For this review, take the finished solid that the model builds, in its own axes (mm). Face numbers are marked on the shaded views. A direction names the side the tool comes from. Give positions to 0.01 mm unless a question says otherwise; leave off trailing zeros. Order: outer loops, then holes, each group sorted by start corner. A loop starts at its lowest first (then second) coordinate and runs counter-clockwise, first axis right, second up. Notation, with made-up numbers: (-33, 82.5) - (3, 82.5) arc R20 cw to (3, 109.5) - close; hole circle Ø9 at (-16.75, 3). An arc over 180 degrees is marked (long way). One line per item, written item: value.
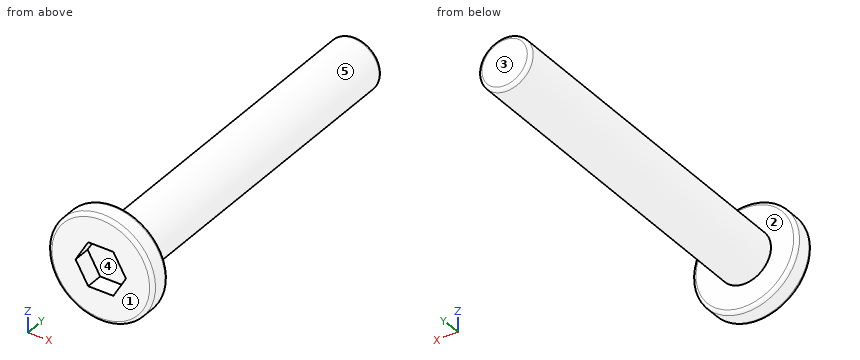
```python
from build123d import *

# Parameters (mm, degrees)
FILLET1_R          = 0.2
CUT_EXTRUDE1_DEPTH = 1


with BuildPart() as part:
    # Sketch2 → Revolve1 (revolve)
    with BuildSketch(Plane.XY, mode=Mode.PRIVATE) as revolve1_sk:
        Polygon((0, 0), (3, 0), (3, 1.2), (1.5, 1.2), (1.5, 21.2), (0, 21.2), align=None)
    revolve(revolve1_sk.sketch.rotate(Axis((0, 73.114266362, 0), (0, -1, 0)), 90), axis=Axis((0, 73.114266362, 0), (0, -1, 0)))

    # Fillet1
    fillet1_edges = [part.edges().sort_by_distance(p)[0] for p in [
        (0, 21.2, -1.5),
        (0, 1.2, -3),
        (0, 0, -3),
    ]]
    fillet(fillet1_edges, radius=FILLET1_R)

    # Sketch3 → Cut-Extrude1 (cut)
    with BuildSketch(Plane.XZ):
        Polygon((1.443375673, 0), (0.721687836, 1.25), (-0.721687836, 1.25), (-1.443375673, 0), (-0.721687836, -1.25), (0.721687836, -1.25), align=None)
    extrude(amount=-CUT_EXTRUDE1_DEPTH, mode=Mode.SUBTRACT)


solid = part.part
```
(1) Draft analysis for pull direction Z (two halves, no side actions). For the marked faces 3, 4 and 5, state which applies: pulls with the +Z half, pulls with the -Z half, needs draft (parallel to the pull), parting line crosses it, or undercut.
Answers below:
face 3: needs draft
face 4: undercut
face 5: parting line crosses it
(2) Take a section at A-A (x = 0). Write out the cut boundary in (y, z).
Answers below:
outline: (0, -2.8) arc R0.2 ccw to (0.2, -3) - (1, -3) arc R0.2 ccw to (1.2, -2.8) - (1.2, -1.5) - (21, -1.5) arc R0.2 ccw to (21.2, -1.3) - (21.2, 1.3) arc R0.2 ccw to (21, 1.5) - (1.2, 1.5) - (1.2, 2.8) arc R0.2 ccw to (1, 3) - (0.2, 3) arc R0.2 ccw to (0, 2.8) - (0, 1.25) - (1, 1.25) - (1, -1.25) - (0, -1.25) - close
(3) Machinability: for the marked faces 1 and 2, which of the approach directions +Z, -Z, +X, -X, +Y, -Y give a long, thin tool a straight path to every point of the face, cutting with its end or side? Answer none if there is none.
Answers below:
face 1: +Z, -Z, +X, -X, -Y
face 2: +Y
(4) For P1, Ø0.5, axis at x = -0.5, y = 0.5, coming from the -Z side; P2, Ø3, axis at x = -1, y = 6, coming from the -Z side; P3, Ø2, axis at x = 0, z = 0, coming from the -Y side, all flat-tipped, find the tip position at first contact; note any pin that passes through.
Answers below:
P1: stops at z = -2.99
P2: stops at z = -1.5
P3: stops at y = 1
(5) Take a section at B-B (y = 4.25). Write out the cut boundary in (x, z).
Answers below:
outline: circle Ø3 at (0, 0)
(6) Wall thickness on line 1 (Y direction, x = 2.5, z = 0.25); line 2 (Y direction, x = 0.25, z = -0.25); line 3 (X direction, y = 12, z = -0.5): over which ranges is each line inside the solid? List them lowest first. Write a range as from..to.
Answers below:
line 1: y = 0..1.2
line 2: y = 1..21.2
line 3: x = -1.41..1.41
